```python
from build123d import *

# Parameters (mm, degrees)
SKETCH1_W                           = 96.210678118
SKETCH1_H                           = 96.210678118
SKETCH1_R                           = 4.25
BODY_EXTRUSION_AND_BOLT_HOLES_DEPTH = 5
SKETCH3_R                           = 10
CENTER_BORE_DEPTH                   = 22.5
SKETCH4_R                           = 40.558917197
SKETCH4_R_2                         = 39.058917197
O_RING_GROOVE_DEPTH                 = 1.5
CUT_EXTRUDE2_START                  = -1.5
SKETCH6_R                           = 40.558917197
SKETCH6_R_2                         = 39.058917197
CUT_EXTRUDE2_DEPTH                  = 1.5


with BuildPart() as part:
    # Sketch1 → body extrusion and bolt holes (new body)
    with BuildSketch(Plane(origin=(0, 0, 0), x_dir=(1, 0, 0), z_dir=(0, 1, 0))):
        Rectangle(SKETCH1_W, SKETCH1_H)
        with Locations(Location((-35.355339059, 35.355339059, 0), (0, 0, 270))):
            Circle(SKETCH1_R, mode=Mode.SUBTRACT)
        with Locations(Location((35.355339059, 35.355339059, 0), (0, 0, 270))):
            Circle(SKETCH1_R, mode=Mode.SUBTRACT)
        with Locations(Location((35.355339059, -35.355339059, 0), (0, 0, 270))):
            Circle(SKETCH1_R, mode=Mode.SUBTRACT)
        with Locations(Location((-35.355339059, -35.355339059, 0), (0, 0, 270))):
            Circle(SKETCH1_R, mode=Mode.SUBTRACT)
    extrude(amount=BODY_EXTRUSION_AND_BOLT_HOLES_DEPTH)

    # Sketch3 → center bore (cut)
    with BuildSketch(Plane(origin=(0, 5, 0), x_dir=(1, 0, 0), z_dir=(0, 1, 0))):
        with Locations(Location((0, 0, 0), (0, 0, 270))):
            Circle(SKETCH3_R)
    extrude(amount=-CENTER_BORE_DEPTH, mode=Mode.SUBTRACT)

    # Sketch4 → o-ring groove (cut)
    with BuildSketch(Plane(origin=(0, 5, 0), x_dir=(1, 0, 0), z_dir=(0, 1, 0))):
        with Locations(Location((0, 0, 0), (0, 0, 270))):
            Circle(SKETCH4_R)
        with Locations(Location((0, 0, 0), (0, 0, 270))):
            Circle(SKETCH4_R_2, mode=Mode.SUBTRACT)
    extrude(amount=-O_RING_GROOVE_DEPTH, mode=Mode.SUBTRACT)

    # Sketch6 → Cut-Extrude2 (cut)
    with BuildSketch(Plane.XZ.offset(CUT_EXTRUDE2_START)):
        with Locations(Location((0, 0, 0), (0, 0, 90))):
            Circle(SKETCH6_R)
        with Locations(Location((0, 0, 0), (0, 0, 90))):
            Circle(SKETCH6_R_2, mode=Mode.SUBTRACT)
    extrude(amount=CUT_EXTRUDE2_DEPTH, mode=Mode.SUBTRACT)


solid = part.part
```
Check sheet for the modelled part. Datum: model origin and axes. Units: mm. A direction names the side the tool comes from. Round coordinates to 2 decimals unless told otherwise and drop trailing zeros. Loops run counter-clockwise (first coordinate to the right, second up) from the corner with the lowest first, then second, coordinate; pieces in that order, holes last. Notation, with made-up numbers: (-17.5, 3) - (14.5, 3) arc R32 ccw to (14.5, 33) - close; hole circle Ø1 at (17.25, 81). An arc over 180 degrees is marked (long way). Answer as a JSON object with one key per item and string values. Group by question number.
Q1. Sectioned sample at A-A, the plane x = 0. Enter the section's corners in (y, z), plus the area to 3 significant figures.
Q2. Sectioned sample at D-D, the plane y = 2.25. Enter the section's corners in (x, z).
Q3. Sectioned sample at C-C, the plane x = -25.5. Enter the section's corners in (y, z).
Q4. Mould release check, pull along Z, two halves, no side actions. Record for faces 1 (the face through (-9.76, 2.54, -2.17)), 2 (the face through (-1, 2, 48.105)), 3 (the face through (42, 5, -1)), 4 (the face through (39.594, 0.76, -8.792)): released by +Z, released by -Z, zero draft, split by the parting line, or undercut.
Q5. Set-up check for faces 5 (the face through (-39.594, 4.26, -8.792)), 6 (the face through (-33.2, 1.5, -21.2)), 7 (the face through (8, 5, 8)): record each of +Z, -Z, +X, -X, +Y, -Y from which the full face is reachable in a straight line by a thin tool's end or side.
Q6. Gauge pin test, flat end, axial feed: P1, Ø7, axis at x = -35.36, z = -35.36, coming from the +Y side. Record the tip position at first contact, or that the pin passes through.
Q7. Scan lines: line 1 along X through (y, z) = (4.4, 0); line 2 along X through (y, z) = (0.25, -5.5); line 3 along Z through (x, y) = (-18.5, 1.2). Record each from-to range of solid material in increasing order. Write a range as [from, to].
Q8. Sectioned sample at B-B, the plane z = 0. Enter the section's corners in (x, y).
Solution:
{
 "1": {"outline": "(0, -48.11) - (5, -48.11) - (5, -40.56) - (3.5, -40.56) - (3.5, -39.06) - (5, -39.06) - (5, -10) - (0, -10) - (0, -39.06) - (1.5, -39.06) - (1.5, -40.56) - (0, -40.56) - close; (0, 10) - (5, 10) - (5, 39.06) - (3.5, 39.06) - (3.5, 40.56) - (5, 40.56) - (5, 48.11) - (0, 48.11) - (0, 40.56) - (1.5, 40.56) - (1.5, 39.06) - (0, 39.06) - close", "area": "372 mm²"},
 "2": {"outline": "(-48.11, -48.11) - (48.11, -48.11) - (48.11, 48.11) - (-48.11, 48.11) - close; hole circle Ø8.5 at (-35.36, -35.36); hole circle Ø8.5 at (-35.36, 35.36); hole circle Ø20 at (0, 0); hole circle Ø8.5 at (35.36, -35.36); hole circle Ø8.5 at (35.36, 35.36)"},
 "3": {"outline": "(0, -48.11) - (5, -48.11) - (5, -31.54) - (3.5, -31.54) - (3.5, -29.59) - (5, -29.59) - (5, 29.59) - (3.5, 29.59) - (3.5, 31.54) - (5, 31.54) - (5, 48.11) - (0, 48.11) - (0, 31.54) - (1.5, 31.54) - (1.5, 29.59) - (0, 29.59) - (0, -29.59) - (1.5, -29.59) - (1.5, -31.54) - (0, -31.54) - close"},
 "4": {"face 1": "undercut", "face 2": "released by +Z", "face 3": "zero draft", "face 4": "undercut"},
 "5": {"face 5": "+Y", "face 6": "-Y", "face 7": "+Z, -Z, +X, -X, +Y"},
 "6": {"P1": "passes through"},
 "7": {"line 1": "x = [-48.11, -40.56], [-39.06, -10], [10, 39.06], [40.56, 48.11]", "line 2": "x = [-48.11, -40.18], [-38.67, -8.35], [8.35, 38.67], [40.18, 48.11]", "line 3": "z = [-48.11, -36.09], [-34.4, 34.4], [36.09, 48.11]"},
 "8": {"outline": "(-48.11, 0) - (-40.56, 0) - (-40.56, 1.5) - (-39.06, 1.5) - (-39.06, 0) - (-10, 0) - (-10, 5) - (-39.06, 5) - (-39.06, 3.5) - (-40.56, 3.5) - (-40.56, 5) - (-48.11, 5) - close; (10, 0) - (39.06, 0) - (39.06, 1.5) - (40.56, 1.5) - (40.56, 0) - (48.11, 0) - (48.11, 5) - (40.56, 5) - (40.56, 3.5) - (39.06, 3.5) - (39.06, 5) - (10, 5) - close"}
}
